Here's how the part is built. I have some questions about the finished solid (model axes, mm). A direction names the side the tool comes from. Give positions to 0.01 mm unless a question says otherwise; leave off trailing zeros. Loops run counter-clockwise (first coordinate to the right, second up) from the corner with the lowest first, then second, coordinate; pieces in that order, holes last. Notation, with made-up numbers: (46, 58.5) - (81, 58.5) arc R35 cw to (81, 90.5) - close; hole circle Ø10 at (19.25, 21). An arc over 180 degrees is marked (long way). Return JSON: item names as keys, results as strings. Group by question number.
(1) If we section it at B-B (z = 2.05): Please give me the cut outline in (x, y), then the cut area to 3 significant figures.
(2) For P1, Ø1.5, axis at y = 50, z = 1.5, coming from the +X side, with a flat end and sliding along its axis, tell me the tip position at first contact or that it passes through.
(3) On a 3-axis mill with a long thin cutter (end or side, diameter ignored), from which of +Z, -Z, +X, -X, +Y, -Y can I reach the whole of each face in a straight line? I mean faces 1 (the flat face through (130, 44, 3)), 2 (the flat face through (0, 45, 3)). Say none if no direction works.
(4) If we section it at C-C (y = 44.5): Please give me the cut outline in (x, z).
(5) If we mould it in two halves opening along X, with no side actions, what happens to faces 3 (the cylindrical face through (131.574, 22.496, 2.958)), 4 (the flat face through (69, 45, 0)), 5 (the flat face through (135, 25, 3))? For each: released by +X, released by -X, zero draft, split by the parting line, or undercut.
(6) I need wall thicknesses on probe 1 along X at (y, z) = (66, 1.75); probe 2 along Y at (x, z) = (10, 4.05); probe 3 along X at (y, z) = (56.5, 4.9). Which ranges of each line are inside material? Lowest first, please. Write a range as [from, to].
(7) If we section it at A-A (x = 10): Please give me the cut outline in (y, z), then the cut area to 3 significant figures.
```python
from build123d import *

# Parameters (mm, degrees)
SKETCH1_R           = 1.65
BOSS_EXTRUDE1_DEPTH = 6


with BuildPart() as part:
    # Sketch1 → Boss-Extrude1 (new body)
    with BuildSketch(Plane.XY):
        Polygon((0, 0), (140, 1.2e-05), (139.99998, 22.000012), (130, 28), (130, 60), (139.99998, 65.999988), (140, 87.999988), (0, 88), align=None)
        with Locations((10, 22)):
            Circle(SKETCH1_R, mode=Mode.SUBTRACT)
        with Locations(Location((130, 66, 0), (0, 0, 180))):
            Circle(SKETCH1_R, mode=Mode.SUBTRACT)
        with Locations((130, 22)):
            Circle(SKETCH1_R, mode=Mode.SUBTRACT)
        with Locations(Location((10, 66, 0), (0, 0, 180))):
            Circle(SKETCH1_R, mode=Mode.SUBTRACT)
    extrude(amount=BOSS_EXTRUDE1_DEPTH)


solid = part.part
```
Values:
{
 "1": {"outline": "(0, 0) - (140, 0) - (140, 22) - (130, 28) - (130, 60) - (140, 66) - (140, 88) - (0, 88) - close; hole circle Ø3.3 at (10, 22); hole circle Ø3.3 at (10, 66); hole circle Ø3.3 at (130, 22); hole circle Ø3.3 at (130, 66)", "area": "11,900 mm2"},
 "2": {"P1": "x = 130"},
 "3": {"face 1": "+Z, -Z, +X", "face 2": "+Z, -Z, -X, +Y, -Y"},
 "4": {"outline": "(0, 0) - (130, 0) - (130, 6) - (0, 6) - close"},
 "5": {"face 3": "undercut", "face 4": "zero draft", "face 5": "released by +X"},
 "6": {"probe 1": "[0, 8.35], [11.65, 128.35], [131.65, 140]", "probe 2": "[0, 20.35], [23.65, 64.35], [67.65, 88]", "probe 3": "[0, 130]"},
 "7": {"outline": "(0, 0) - (20.35, 0) - (20.35, 6) - (0, 6) - close; (23.65, 0) - (64.35, 0) - (64.35, 6) - (23.65, 6) - close; (67.65, 0) - (88, 0) - (88, 6) - (67.65, 6) - close", "area": "488 mm2"}
}
